from build123d import *

# Parameters (mm, degrees)
SKETCH_1_R               = 10
EXTRUDE_1_DEPTH          = 12
SKETCH_2_R               = 11
EXTRUDE_2_DEPTH          = 1
CUT_EXTRUDE_1_DEPTH      = 21.273134933
CUT_EXTRUDE_1_DEPTH_BACK = 6
SKETCH_3_R               = 5
SKETCH_3_R_2             = 3.5
EXTRUDE_START            = 6
SKETCH_5_R               = 3.5
EXTRUDE_3_DEPTH          = 6
SHELL_1_T                = -2
FILLET_1_R               = 3


with BuildPart() as part:
    # ｽｹｯﾁ1 → ﾎﾞｽ - 押し出し1 (new body)
    with BuildSketch(Plane(origin=(0, 0, 0), x_dir=(1, 0, 0), z_dir=(0, 1, 0))):
        with Locations(Location((0, 0, 0), (0, 0, 270))):
            Circle(SKETCH_1_R)
    extrude(amount=EXTRUDE_1_DEPTH)

    # ｽｹｯﾁ2 → ﾎﾞｽ - 押し出し2 (add)
    with BuildSketch(Plane.XZ):
        with Locations(Location((0, 0, 0), (0, 0, 270))):
            Circle(SKETCH_2_R)
    extrude(amount=EXTRUDE_2_DEPTH)

    # ｽｹｯﾁ3 → ｶｯﾄ - 押し出し1 (cut, two sides: drawn at the far end of the back side and taken through both)
    with BuildSketch(Plane.XZ.offset(1).offset(-CUT_EXTRUDE_1_DEPTH_BACK)):
        with Locations(Location((0, 0, 0), (0, 0, 90))):
            Circle(SKETCH_3_R)
        with Locations(Location((0, 0, 0), (0, 0, 90))):
            Circle(SKETCH_3_R_2, mode=Mode.SUBTRACT)
    extrude(amount=CUT_EXTRUDE_1_DEPTH + CUT_EXTRUDE_1_DEPTH_BACK, mode=Mode.SUBTRACT)

    # ｽｹｯﾁ5 → ﾎﾞｽ - 押し出し3 (add)
    with BuildSketch(Plane.XZ.offset(1).offset(EXTRUDE_START)):
        with Locations(Location((0, 0, 0), (0, 0, 90))):
            Circle(SKETCH_5_R)
    extrude(amount=-EXTRUDE_3_DEPTH)

    # ｼｪﾙ1
    shell_1_openings = [part.faces().sort_by_distance(p)[0] for p in [
        (0, 12, 0),
    ]]
    offset(amount=SHELL_1_T, openings=shell_1_openings, kind=Kind.INTERSECTION)

    # ﾌｨﾚｯﾄ1
    fillet_1_edges = [part.edges().sort_by_distance(p)[0] for p in [
        (0, 7, -7),
    ]]
    fillet(fillet_1_edges, radius=FILLET_1_R)


solid = part.part
For this review, take the finished solid that the model builds, in its own axes (mm). A direction names the side the tool comes from. Round coordinates to 2 decimals unless told otherwise and drop trailing zeros. Order: outer loops, then holes, each group sorted by start corner. A loop starts at its lowest first (then second) coordinate and runs counter-clockwise, first axis right, second up. Notation, with made-up numbers: M 22,-21 L 75,-21 A27 ccw 75,10 Z; hole C 80,-20.5 d7. An arc over 180 degrees is marked long. Use a Markdown table: item, result. Add a question column.
Item 1: Tool access review of faces 1 (the cylindrical face through (3.417, -1.084, -0.759)), 2 (the flat face through (8.2, 12, 0)), 3 (the flat face through (-10, 0, -2)): name each direction out of +Z, -Z, +X, -X, +Y, -Y from which nothing blocks a thin tool from reaching the whole face with its end or side.
Item 2: Add section D-D, the plane y = 10. Give the boundary of the cut face in (x, z).
Item 3: Add section A-A, the plane y = 1.5. Give the boundary of the cut face in (x, z), then the cut area to 3 significant figures.
Item 4: To check wall thickness, follow line 1 along X through (y, z) = (2.8, 0); line 2 along X through (y, z) = (0.65, 0); line 3 along Y through (x, z) = (1.25, -9.5). State the ranges of each line that lie inside material, in increasing order.
Item 5: Insertion check: pin 1 (5 mm diameter, centred on y = 3.5, z = 6, fed in from -X); pin 2 (4 mm diameter, centred on x = 0, z = 0, fed in from +Y); pin 3 (4 mm diameter, centred on x = -7, y = -2, fed in from -Z); pin 4 (1 mm diameter, centred on x = -4.5, y = -2.5, fed in from -Z). Each pin has a flat end and moves straight along its axis. Give the tip position at first contact, or say it passes through.
Item 6: Mouldability with a two-part tool opening along X and no side actions: class faces 4 (the cylindrical face through (-10.74, -0.49, 2.38)), 5 (the flat face through (0, -7, 0)), 6 (the flat face through (3.3, 5, 2.2)) as released by +X, released by -X, zero draft, split by the parting line, or undercut.
Geometry results:
| question | item | result |
|---|---|---|
| 1 | face 1 | -Y |
| 1 | face 2 | +Z, -Z, +X, -X, +Y |
| 1 | face 3 | +Y |
| 2 | outline | C 0,0 d20; hole C 0,0 d16 |
| 3 | outline | C 0,0 d20; C 0,0 d14; C 0,0 d7; hole C 0,0 d16; hole C 0,0 d10; hole C 0,0 d3 |
| 3 | area | 220 mm² |
| 4 | line 1 | x = -10 to -8, -7 to -5, -3.5 to -1.5, 1.5 to 3.5, 5 to 7, 8 to 10 |
| 4 | line 2 | x = -10 to -5, -3.5 to -1.5, 1.5 to 3.5, 5 to 10 |
| 4 | line 3 | y = -1 to 12 |
| 5 | pin 1 | stops at x = -9.37 |
| 5 | pin 2 | stops at y = 7 |
| 5 | pin 3 | stops at z = -9.66 |
| 5 | pin 4 | passes through |
| 6 | face 4 | split by the parting line |
| 6 | face 5 | zero draft |
| 6 | face 6 | undercut |
